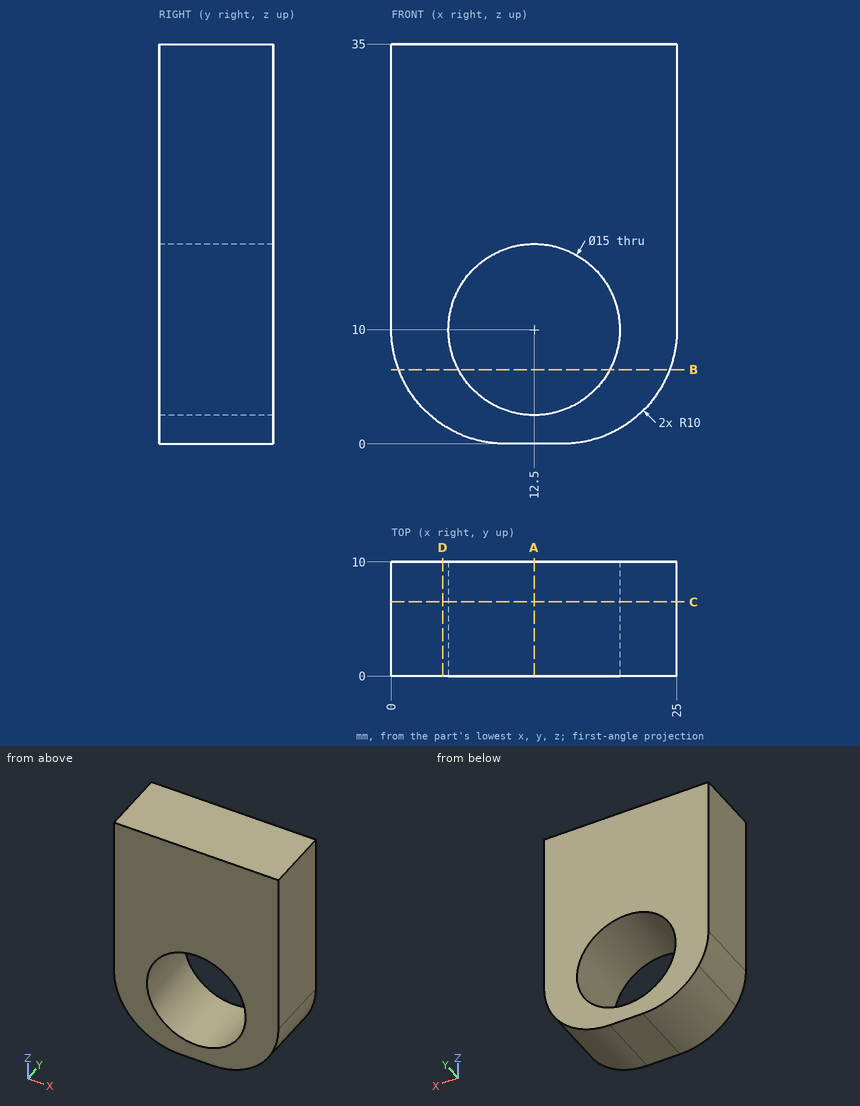
Answer from the drawing. Dimensions are ordinates in mm from the lowest x, y and z of the part. Round coordinates to 2 decimals unless told otherwise and drop trailing zeros. Order: outer loops, then holes, each group sorted by start corner. A loop starts at its lowest first (then second) coordinate and runs counter-clockwise, first axis right, second up.
1) The part is cut by section B-B on z = 6.5. Write down the section's boundary in (x, y).
2) The part is cut by section A-A on x = 12.5. Write down the section's boundary in (y, z).
3) The part is cut by section D-D on x = 4.5. Write down the section's boundary in (y, z), plus the area to 3 significant figures.
4) The part is cut by section C-C on y = 6.5. Write down the section's boundary in (x, z).
5) A flat-ended cylindrical pin translates along its axis: pin 1 (5 mm diameter, centred on x = 6, y = 5.5, fed in from -Z). Find the tip coordinate at first contact, or state that the pin passes through.
6) Straight lines are drawn through the part: L1, parallel to X at y = 7.5, z = 10; L2, parallel to X at y = 9.5, z = 5; L3, parallel to Z at x = 22, y = 3.5. For each, find the intervals that lie inside material, in ascending order.
Resolved:
1. outline: (0.63, 0) - (5.87, 0) - (5.87, 10) - (0.63, 10) - close; (19.13, 0) - (24.37, 0) - (24.37, 10) - (19.13, 10) - close
2. outline: (0, 0) - (10, 0) - (10, 2.5) - (0, 2.5) - close; (0, 17.5) - (10, 17.5) - (10, 35) - (0, 35) - close
3. outline: (0, 1.65) - (10, 1.65) - (10, 35) - (0, 35) - close
3. area: 334 mm2
4. outline: (0, 10) arc R10 ccw to (10, 0) - (15, 0) arc R10 ccw to (25, 10) - (25, 35) - (0, 35) - close; hole circle Ø15 at (12.5, 10)
5. pin 1: stops at z = 0.11
6. L1: x = 0 to 5, 20 to 25
6. L2: x = 1.34 to 6.91, 18.09 to 23.66
6. L3: z = 2.86 to 35
